Check sheet for the modelled part. Datum: model origin and axes. Units: mm. Give positions to 0.01 mm unless a question says otherwise; leave off trailing zeros. Loops run counter-clockwise (first coordinate to the right, second up) from the corner with the lowest first, then second, coordinate; pieces in that order, holes last. Notation, with made-up numbers: (30, 21) - (87, 21) arc R35 ccw to (87, 56) - close; hole circle Ø8 at (-21.75, 81). An arc over 180 degrees is marked (long way). Answer in a Markdown table with one row per item. Add a question column.
(1) Thickness scan on L1, parallel to Y at x = -5.5, z = 13.5; L2, parallel to Y at x = -2.5, z = 7; L3, parallel to X at y = 1.5, z = 17.25. Record the ranges inside material, lowest first.
(2) Sectioned sample at A-A on z = 7.25. Enter the section's corners in (x, y), then the cut area to 3 significant figures.
(3) Go/stop test with flat-tipped pins: P1, Ø4, axis at x = 5, z = 3, coming from the +Y side; P2, Ø2, axis at x = -3.5, z = 4.5, coming from the +Y side; P3, Ø1, axis at y = -5.5, z = 12.5, coming from the -X side. Record where each tip stops, or that it passes through.
(4) Sectioned sample at B-B on y = 3.25. Enter the section's corners in (x, z), then the cut area to 3 significant figures.
from build123d import *

# Parameters (mm, degrees)
F1_DEPTH = 19.05


with BuildPart() as f1:
    # F0 (on Top) → F1 (new body)
    with BuildSketch(Plane.XY):
        Polygon((5.659421, 4.75631), (3.912648, 6.272377), (1.782879, 7.17446), (-0.521412, 7.374257), (-2.774663, 6.85221), (-4.75631, 5.659421), (-6.272377, 3.912648), (-7.17446, 1.782879), (-7.374257, -0.521412), (-6.85221, -2.774663), (-5.659421, -4.75631), (-3.912648, -6.272377), (-1.782879, -7.17446), (0.521412, -7.374257), (2.774663, -6.85221), (4.75631, -5.659421), (6.272377, -3.912648), (7.17446, -1.782879), (7.374257, 0.521412), (6.85221, 2.774663), align=None)
    extrude(amount=F1_DEPTH)


solid = f1.part
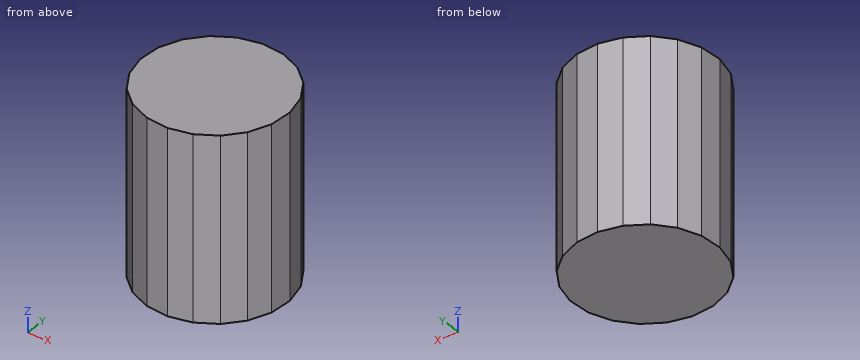
Reply:
| question | item | result |
|---|---|---|
| 1 | L1 | -4.89 to 4.8 |
| 1 | L2 | -6.87 to 6.92 |
| 1 | L3 | -7.2 to 7.15 |
| 2 | outline | (-7.37, -0.52) - (-6.85, -2.77) - (-5.66, -4.76) - (-3.91, -6.27) - (-1.78, -7.17) - (0.52, -7.37) - (2.77, -6.85) - (4.76, -5.66) - (6.27, -3.91) - (7.17, -1.78) - (7.37, 0.52) - (6.85, 2.77) - (5.66, 4.76) - (3.91, 6.27) - (1.78, 7.17) - (-0.52, 7.37) - (-2.77, 6.85) - (-4.76, 5.66) - (-6.27, 3.91) - (-7.17, 1.78) - close |
| 2 | area | 169 mm^2 |
| 3 | P1 | y = 6.66 |
| 3 | P2 | y = 6.92 |
| 3 | P3 | x = -5.38 |
| 4 | outline | (-6.55, 0) - (6.57, 0) - (6.57, 19.05) - (-6.55, 19.05) - close |
| 4 | area | 250 mm^2 |
